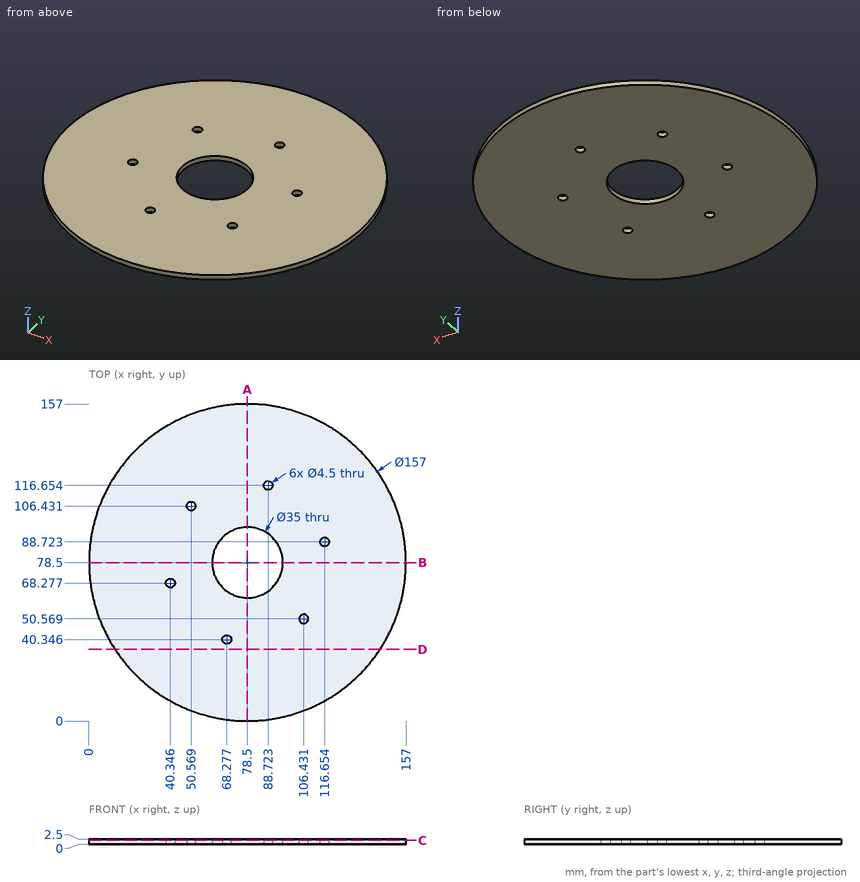
Answer from the drawing. Dimensions are ordinates in mm from the lowest x, y and z of the part. Coordinates: 2 decimals unless noted, no trailing zeros. Order: outer loops, then holes, each group sorted by start corner. A loop starts at its lowest first (then second) coordinate and runs counter-clockwise, first axis right, second up. Notation, with made-up numbers: (-17, 32.5) - (27, 32.5) arc R19 ccw to (27, 48.5) - close; hole circle Ø2 at (30, -9.75). An arc over 180 degrees is marked (long way). Answer as a JSON object with one key per item and string values. Group by question number.
Item 1: Section D-D (y = 35.5) is taken. Give the vertices of the cut face in (x, z) (1 decimal).
Item 2: Section C-C (z = 1.8) is taken. Give the vertices of the cut face in (x, y), plus the area to 3 significant figures.
Item 3: Consider probe 1 along Y at (x, z) = (78.5, 0.7); probe 2 along Y at (x, z) = (90, 1.25) (1 decimal); probe 3 along Y at (x, z) = (70, 1.25) (1 decimal). Determine where each line is inside the solid, lowest interval first. Write a range as from..to.
Item 4: A flat-ended cylindrical pin translates along its axis: P1, Ø1, axis at x = 49, z = 0.5, coming from the -Y side. Find the tip coordinate at first contact, or state that the pin passes through.
Item 5: Section A-A (x = 78.5) is taken. Give the vertices of the cut face in (y, z), plus the area to 3 significant figures.
Results are:
{
 "1": {"outline": "(12.8, 0) - (144.2, 0) - (144.2, 2.5) - (12.8, 2.5) - close"},
 "2": {"outline": "circle Ø157 at (78.5, 78.5); hole circle Ø4.5 at (40.35, 68.28); hole circle Ø4.5 at (50.57, 106.43); hole circle Ø35 at (78.5, 78.5); hole circle Ø4.5 at (68.28, 40.35); hole circle Ø4.5 at (88.72, 116.65); hole circle Ø4.5 at (106.43, 50.57); hole circle Ø4.5 at (116.65, 88.72)", "area": "18,300 mm^2"},
 "3": {"probe 1": "y = 0..61, 96..157", "probe 2": "y = 0.8..65.3, 91.7..114.8, 118.5..156.2", "probe 3": "y = 0.5..38.9, 41.8..63.2, 93.8..156.5"},
 "4": {"P1": "stops at y = 5.55"},
 "5": {"outline": "(0, 0) - (61, 0) - (61, 2.5) - (0, 2.5) - close; (96, 0) - (157, 0) - (157, 2.5) - (96, 2.5) - close", "area": "305 mm^2"}
}
